Verification items for this drawing (mm, ordinates from the low corner). A direction names the side the tool comes from. Round coordinates to 2 decimals unless told otherwise and drop trailing zeros. Order: outer loops, then holes, each group sorted by start corner. A loop starts at its lowest first (then second) coordinate and runs counter-clockwise, first axis right, second up. Notation, with made-up numbers: (88.5, 84.5) -> (112.5, 84.5) arc R30 cw to (112.5, 112.5) -> close; hole circle Ø1 at (33, -23). An arc over 180 degrees is marked (long way). Return JSON: item names as keys, results as strings. Group by question number.
Item 1: Draft check along X on the marked faces 4, 5 and 6. Enter one of: pulls with the +X half, pulls with the -X half, needs draft (parallel to the pull), parting line crosses it, or undercut.
Item 2: Sectioned sample at D-D on x = 13.5. Record the cut outline in (y, z), plus the area to 3 significant figures.
Item 3: Sectioned sample at B-B on x = 5.5. Record the cut outline in (y, z).
Item 4: Depth check by flat-ended pin: pin 1 Ø5 at (y, z) = (10, 12) entering from -X; pin 2 Ø0.6 at (x, z) = (0.5, 22.5) entering from -Y. Enter the tip coordinate at first touch or a pass-through.
Item 5: Access from +Z, -Z, +X, -X, +Y, -Y to the whole of each face (thin tool, end or side, straight path). Record for the marked faces 1, 2 and 3.
Item 6: Sectioned sample at A-A on x = 10. Record the cut outline in (y, z).
Item 7: Scan lines: probe 1 along X at (y, z) = (5, 38); probe 2 along X at (y, z) = (17.75, 44); probe 3 along X at (y, z) = (4.5, 13.5). Record each from-to range of solid material in increasing order. Write a range as from..to.
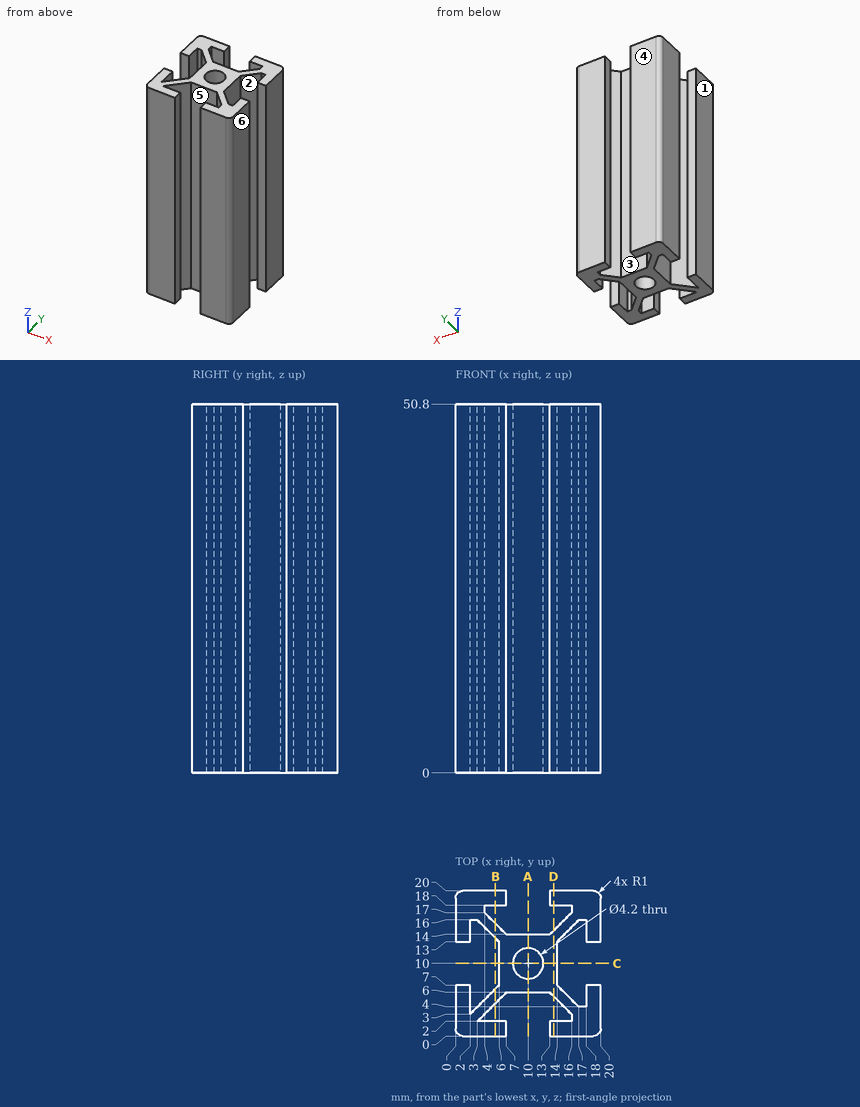
Recorded:
{
 "1": {"face 4": "needs draft", "face 5": "undercut", "face 6": "pulls with the +X half"},
 "2": {"outline": "(0, 0) -> (2, 0) -> (2, 50.8) -> (0, 50.8) -> close; (5.5, 0) -> (14.5, 0) -> (14.5, 50.8) -> (5.5, 50.8) -> close; (18, 0) -> (20, 0) -> (20, 50.8) -> (18, 50.8) -> close", "area": "660 mm²"},
 "3": {"outline": "(0, 0) -> (2, 0) -> (2, 50.8) -> (0, 50.8) -> close; (4.5, 0) -> (6.5, 0) -> (6.5, 50.8) -> (4.5, 50.8) -> close; (13.5, 0) -> (15.5, 0) -> (15.5, 50.8) -> (13.5, 50.8) -> close; (18, 0) -> (20, 0) -> (20, 50.8) -> (18, 50.8) -> close"},
 "4": {"pin 1": "x = 6", "pin 2": "y = 0.02"},
 "5": {"face 1": "+Z, -Z, -X, +Y, -Y", "face 2": "+Z, -Z", "face 3": "+Z, -Z, +Y"},
 "6": {"outline": "(6, 0) -> (7.9, 0) -> (7.9, 50.8) -> (6, 50.8) -> close; (12.1, 0) -> (14, 0) -> (14, 50.8) -> (12.1, 50.8) -> close"},
 "7": {"probe 1": "0..2, 4..6, 14..16, 18..20", "probe 2": "0..4, 16..20", "probe 3": "0..2, 3.5..5.5, 14.5..16.5, 18..20"}
}
